Could you check a few things on this model? Use its own coordinates, in mm. Round coordinates to 2 decimals unless told otherwise and drop trailing zeros. Loops run counter-clockwise (first coordinate to the right, second up) from the corner with the lowest first, then second, coordinate; pieces in that order, holes last. Notation, with made-up numbers: (25.5, -28) -> (78.5, -28) arc R19 ccw to (78.5, -6) -> close; hole circle Ø7 at (71, 68.5). An arc over 180 degrees is marked (long way). One line per item, written item: value.
from build123d import *

# Parameters (mm, degrees)
BOSS_EXTRUDE1_DEPTH      = 1.0541
BOSS_EXTRUDE1_DEPTH_BACK = 1.0541
SKETCH3_R                = 12.7
SKETCH3_R_2              = 5.5626
FILLET1_R                = 0.21082


with BuildPart() as part:
    # Sketch3 → Boss-Extrude1 (new, two sides: drawn at the far end of the back side and taken through both)
    with BuildSketch(Plane.XY.offset(-BOSS_EXTRUDE1_DEPTH_BACK)):
        Circle(SKETCH3_R)
        Circle(SKETCH3_R_2, mode=Mode.SUBTRACT)
    extrude(amount=BOSS_EXTRUDE1_DEPTH + BOSS_EXTRUDE1_DEPTH_BACK)

    # Fillet1
    fillet1_edges = [part.edges().sort_by_distance(p)[0] for p in [
        (-12.7, 0, -1.0541),
        (-5.5626, 0, -1.0541),
        (-12.7, 0, 1.0541),
        (-5.5626, 0, 1.0541),
    ]]
    fillet(fillet1_edges, radius=FILLET1_R)


solid = part.part
(1) If we section it at A-A, the plane x = 0: Please give me the cut outline in (y, z), then the cut area to 3 significant figures.
Recorded:
outline: (-12.7, -0.84) arc R0.21 ccw to (-12.49, -1.05) -> (-5.77, -1.05) arc R0.21 ccw to (-5.56, -0.84) -> (-5.56, 0.84) arc R0.21 ccw to (-5.77, 1.05) -> (-12.49, 1.05) arc R0.21 ccw to (-12.7, 0.84) -> close; (5.56, -0.84) arc R0.21 ccw to (5.77, -1.05) -> (12.49, -1.05) arc R0.21 ccw to (12.7, -0.84) -> (12.7, 0.84) arc R0.21 ccw to (12.49, 1.05) -> (5.77, 1.05) arc R0.21 ccw to (5.56, 0.84) -> close
area: 30.0 mm²
(2) If we section it at C-C, the plane z = 0.25: Please give me the cut outline in (x, y), then the cut area to 3 significant figures.
Recorded:
outline: circle Ø25.4 at (0, 0); hole circle Ø11.13 at (0, 0)
area: 409 mm²
(3) If I drill on L1, parallel to Y at x = 0, z = -0.15; L2, parallel to Y at x = -1.25, z = -0.35; L3, parallel to X at y = -3, z = 0.25, over which ranges is the centre line in solid material (lowest first)?
Recorded:
L1: -12.7 to -5.56, 5.56 to 12.7
L2: -12.64 to -5.42, 5.42 to 12.64
L3: -12.34 to -4.68, 4.68 to 12.34
(4) Thinking about a two-plate mould opening in Y: for faces 1 (the face through (2.6, -5.4, 1.054)), 2 (the face through (5.306, 1.671, -0.012)), 3 (the face through (-2.75, -12.4, -0.01)), which applies, released by +Y, released by -Y, zero draft, split by the parting line, or undercut?
Recorded:
face 1: zero draft
face 2: undercut
face 3: split by the parting line
(5) I'm going to push flat-ended pins straight in: pin 1 Ø1 at (x, z) = (7, 0) entering from -Y; pin 2 Ø6 at (x, y) = (2.5, 1) entering from -Z. Where does each tip first touch, or does it pass through?
Recorded:
pin 1: y = -10.91
pin 2: z = -1.04
